from build123d import *

# Parameters (mm, degrees)
SKETCH_1_W          = 30
SKETCH_1_H          = 20
EXTRUDE_1_DEPTH     = 5
SKETCH_2_W          = 15
SKETCH_2_H          = 10
CUT_EXTRUDE_1_DEPTH = 19.708286934


with BuildPart() as part:
    # 草图1 → 凸台-拉伸1 (new, symmetric)
    with BuildSketch(Plane(origin=(0, 0, 0), x_dir=(1, 0, 0), z_dir=(0, 1, 0))):
        Rectangle(SKETCH_1_W, SKETCH_1_H)
    extrude(amount=EXTRUDE_1_DEPTH, both=True)

    # 草图2 → 切除-拉伸1 (cut, through all)
    with BuildSketch(Plane(origin=(0, 0, 0), x_dir=(1, 0, 0), z_dir=(0, 1, 0))):
        with Locations((7.5, 5)):
            Rectangle(SKETCH_2_W, SKETCH_2_H)
    extrude(amount=CUT_EXTRUDE_1_DEPTH, mode=Mode.SUBTRACT)


solid = part.part
Geometry check sheet. Reference: the model listing, model coordinates, mm. A direction names the side the tool comes from. Give positions to 0.01 mm unless a question says otherwise; leave off trailing zeros. Write each loop counter-clockwise with the first axis right and the second up, starting at its lowest first coordinate (ties: lowest second). Pieces come first, ordered by that corner, then holes.
1) Thickness scan on line 1 (Y direction, x = 9.5, z = -6.75); line 2 (X direction, y = 0.25, z = -7.75); line 3 (Z direction, x = 5, y = 3.75). Record the ranges inside material, lowest first.
Values follow:
line 1: y = -5 to 0
line 2: x = -15 to 0
line 3: z = 0 to 10
2) Set-up check for faces 1 (the face through (-4, -1, -10)), 2 (the face through (7, 2, 0)): record each of +Z, -Z, +X, -X, +Y, -Y from which the full face is reachable in a straight line by a thin tool's end or side.
Values follow:
face 1: -Z, +X, -X, +Y, -Y
face 2: -Z, +X, +Y
3) Go/stop test with flat-tipped pins: pin 1 Ø1.5 at (x, y) = (5, 3.5) entering from -Z; pin 2 Ø4 at (y, z) = (3.5, -5.5) entering from +X; pin 3 Ø11 at (x, z) = (5, -4) entering from +Y. Record where each tip stops, or that it passes through.
Values follow:
pin 1: stops at z = 0
pin 2: stops at x = 0
pin 3: stops at y = 5
4) Cross-section at B-B (y = 1.5). Record the boundary of the cut face in (x, z).
Values follow:
outline: (-15, -10) - (0, -10) - (0, 0) - (15, 0) - (15, 10) - (-15, 10) - close
5) Cross-section at A-A (x = 4). Record the boundary of the cut face in (y, z).
Values follow:
outline: (-5, -10) - (0, -10) - (0, 0) - (5, 0) - (5, 10) - (-5, 10) - close
